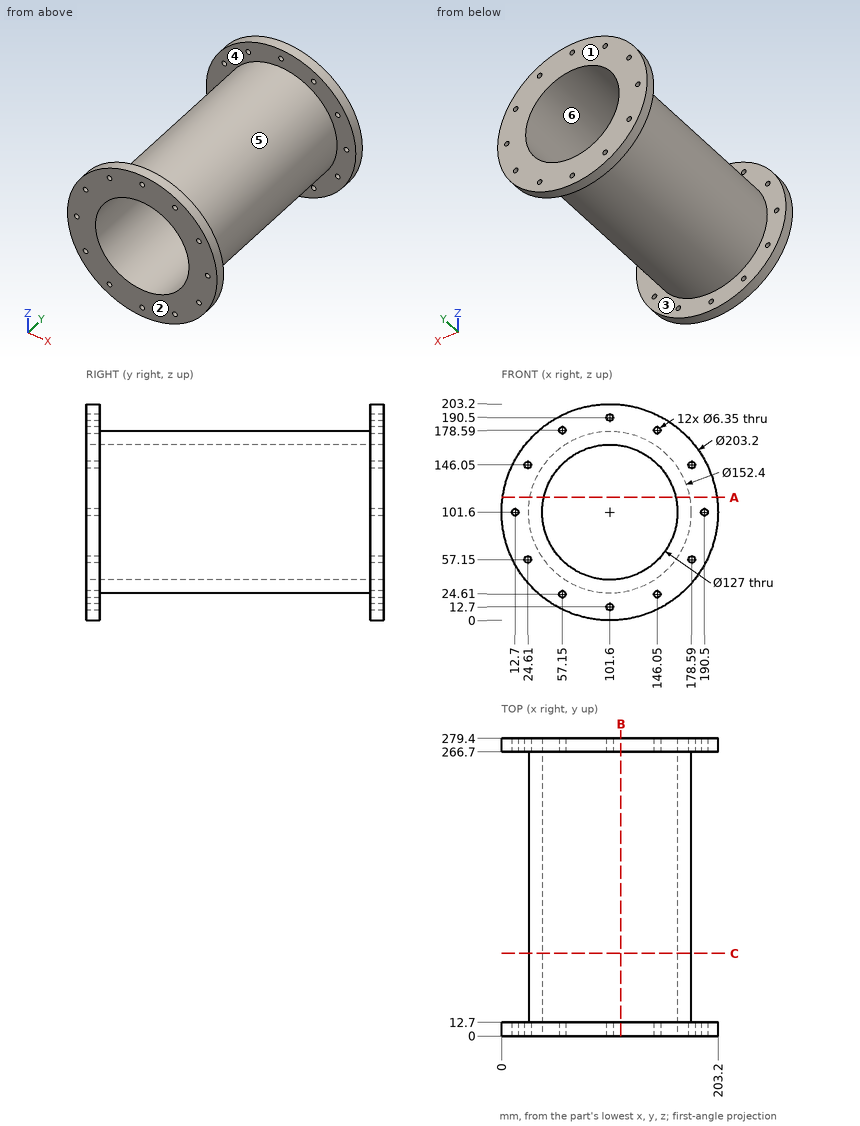
Geometry check sheet. Reference: drawing and pictorial views, mm from the part's lowest x, y, z. A direction names the side the tool comes from. Coordinates: 2 decimals unless noted, no trailing zeros. Write each loop counter-clockwise with the first axis right and the second up, starting at its lowest first coordinate (ties: lowest second). Pieces come first, ordered by that corner, then holes. Notation, with made-up numbers: (81.5, 54.5) -> (109.5, 54.5) arc R18 cw to (109.5, 80.5) -> close; hole circle Ø8 at (84.5, -32). An arc over 180 degrees is marked (long way). Use a Markdown table: item, result.
1. Sectioned sample at A-A (z = 115.5). Enter the section's corners in (x, y) (1 decimal).
Reported:
| item | result |
|---|---|
| outline | (1, 0) -> (39.6, 0) -> (39.6, 279.4) -> (1, 279.4) -> (1, 266.7) -> (26.7, 266.7) -> (26.7, 12.7) -> (1, 12.7) -> close; (163.6, 0) -> (202.2, 0) -> (202.2, 12.7) -> (176.5, 12.7) -> (176.5, 266.7) -> (202.2, 266.7) -> (202.2, 279.4) -> (163.6, 279.4) -> close |
2. Go/stop test with flat-tipped pins: pin 1 Ø5 at (y, z) = (47.5, 134.5) entering from +X; pin 2 Ø5.5 at (x, z) = (101.6, 12.7) entering from +Y; pin 3 Ø3 at (x, y) = (38, 175.5) entering from -Z; pin 4 Ø8.5 at (x, z) = (146.05, 178.59) entering from +Y. Record where each tip stops, or that it passes through.
Reported:
| item | result |
|---|---|
| pin 1 | stops at x = 171.47 |
| pin 2 | passes through |
| pin 3 | stops at z = 57.44 |
| pin 4 | stops at y = 279.4 |
3. Release check for a two-part mould opening along Y. For the marked faces 1, 2, 3 and 4 record: pulls with the +Y half, pulls with the -Y half, needs draft (parallel to the pull), parting line crosses it, or undercut.
Reported:
| item | result |
|---|---|
| face 1 | pulls with the +Y half |
| face 2 | pulls with the -Y half |
| face 3 | undercut |
| face 4 | undercut |
4. Tool access check on the marked faces 5 and 6. Record the directions out of +Z, -Z, +X, -X, +Y, -Y that give a thin tool (end or side, any length) a straight path to the whole face; none if there is none.
Reported:
| item | result |
|---|---|
| face 5 | none |
| face 6 | +Y, -Y |
5. Scan lines: line 1 along X through (y, z) = (3, 101); line 2 along Y through (x, z) = (147.5, 187); line 3 along X through (y, z) = (149, 135) (1 decimal). Record each from-to range of solid material in increasing order.
Reported:
| item | result |
|---|---|
| line 1 | x = 0 to 9.58, 15.82 to 38.1, 165.1 to 187.38, 193.62 to 203.2 |
| line 2 | y = 0 to 12.7, 266.7 to 279.4 |
| line 3 | x = 33.1 to 47.6, 155.6 to 170.1 |
6. Sectioned sample at C-C (y = 77.5). Enter the section's corners in (x, z), plus the area to 3 significant figures.
Reported:
| item | result |
|---|---|
| outline | circle Ø152.4 at (101.6, 101.6); hole circle Ø127 at (101.6, 101.6) |
| area | 5,570 mm2 |
7. Sectioned sample at B-B (x = 112). Enter the section's corners in (y, z).
Reported:
| item | result |
|---|---|
| outline | (0, 0.53) -> (12.7, 0.53) -> (12.7, 26.11) -> (266.7, 26.11) -> (266.7, 0.53) -> (279.4, 0.53) -> (279.4, 38.96) -> (0, 38.96) -> close; (0, 164.24) -> (279.4, 164.24) -> (279.4, 202.67) -> (266.7, 202.67) -> (266.7, 177.09) -> (12.7, 177.09) -> (12.7, 202.67) -> (0, 202.67) -> close |
